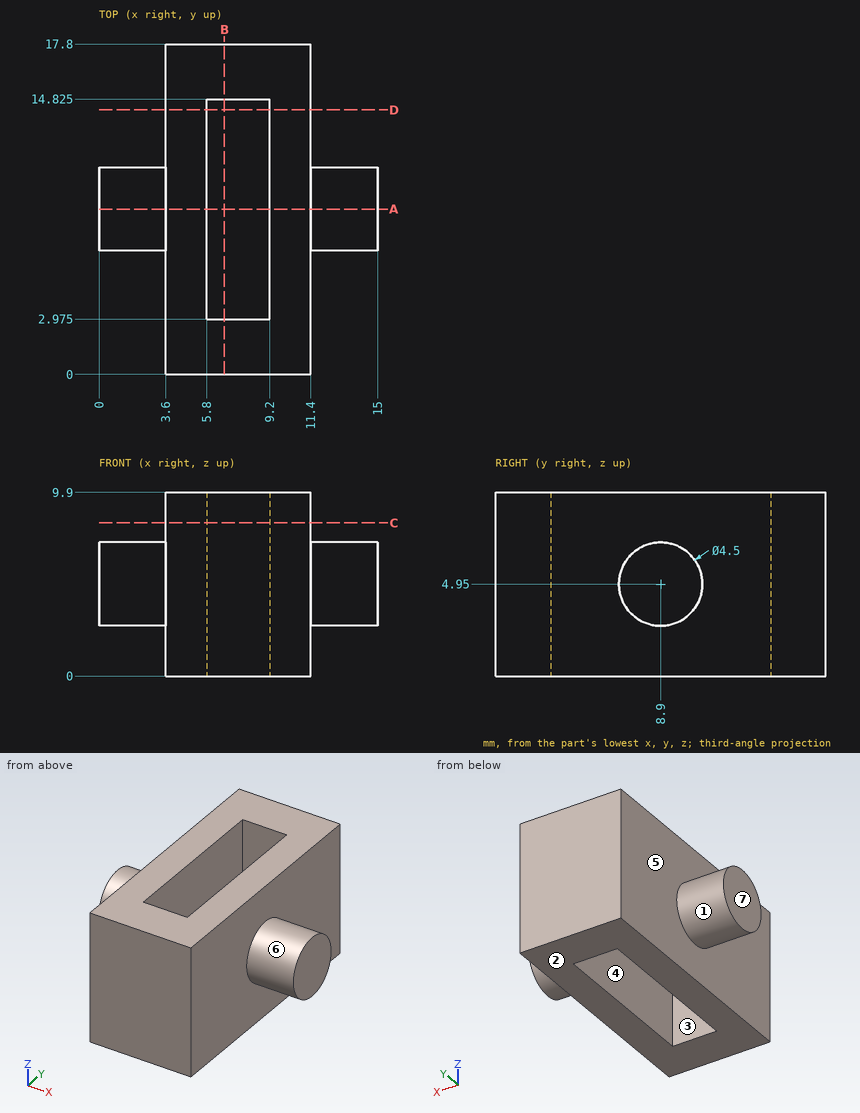
Job drawing, mm, ordinate dimensions from the low corner. One solid piece. A direction names the side the tool comes from. Coordinates: 2 decimals unless noted, no trailing zeros. Loops run counter-clockwise (first coordinate to the right, second up) from the corner with the lowest first, then second, coordinate; pieces in that order, holes last. Notation, with made-up numbers: (59, -7) - (117, -7) arc R22 ccw to (117, 19) - close; hole circle Ø9 at (21.25, -24.5). An arc over 180 degrees is marked (long way). Write item = value, one per line. Start each with the question number.
Q1. Cut at D-D, the plane y = 14.25. List the corners of the cut face in (x, z).
Q2. Cut at B-B, the plane x = 6.75. List the corners of the cut face in (y, z) (3 decimals).
Q3. Pull direction Y, two halves, no side cores. Call the marked faces 1, 2 and 3: pulls with the +Y half, pulls with the -Y half, needs draft (parallel to the pull), parting line crosses it, or undercut.
Q4. Cut at A-A, the plane y = 8.9. List the corners of the cut face in (x, z).
Q5. Flat gauge pins, fed straight in: pin 1 Ø1.5 at (y, z) = (5, 8) entering from +X; pin 2 Ø1 at (y, z) = (9.5, 8.5) entering from -X. Where does each tip first touch, or does it go through?
Q6. Which spindle directions (+Z, -Z, +X, -X, +Y, -Y) get a long thin tool onto all of the face, cutting with end or side? Do the marked faces 4, 5, 6 and 7. Say none if no direction does.
Q7. Cut at C-C, the plane z = 8.25. List the corners of the cut face in (x, y) (3 decimals), then the cut area to 4 significant figures.
Q8. Drill centre lines: L1, parallel to Y at x = 7.5, z = 5.25 (3 decimals); L2, parallel to X at y = 8.5, z = 7; L3, parallel to X at y = 14.75, z = 9.75. Where is each one in solid material? Low to high.
Computed:
q1.outline = (3.6, 0) - (5.8, 0) - (5.8, 9.9) - (3.6, 9.9) - close; (9.2, 0) - (11.4, 0) - (11.4, 9.9) - (9.2, 9.9) - close
q2.outline = (0, 0) - (2.975, 0) - (2.975, 9.9) - (0, 9.9) - close; (14.825, 0) - (17.8, 0) - (17.8, 9.9) - (14.825, 9.9) - close
q3.face_1 = parting line crosses it
q3.face_2 = needs draft
q3.face_3 = undercut
q4.outline = (0, 2.7) - (3.6, 2.7) - (3.6, 0) - (5.8, 0) - (5.8, 9.9) - (3.6, 9.9) - (3.6, 7.2) - (0, 7.2) - close; (9.2, 0) - (11.4, 0) - (11.4, 2.7) - (15, 2.7) - (15, 7.2) - (11.4, 7.2) - (11.4, 9.9) - (9.2, 9.9) - close
q5.pin_1 = 11.4
q5.pin_2 = 3.6
q6.face_4 = +Z, -Z
q6.face_5 = -X
q6.face_6 = +X
q6.face_7 = +Z, -Z, -X, +Y, -Y
q7.outline = (3.6, 0) - (11.4, 0) - (11.4, 17.8) - (3.6, 17.8) - close; hole (5.8, 2.975) - (9.2, 2.975) - (9.2, 14.825) - (5.8, 14.825) - close
q7.area = 98.55 mm²
q8.L1 = 0 to 2.975, 14.825 to 17.8
q8.L2 = 0 to 5.8, 9.2 to 15
q8.L3 = 3.6 to 5.8, 9.2 to 11.4
